from build123d import *

# Parameters (mm, degrees)
F0_R     = 5
F1_DEPTH = 8
F2_W     = 70
F2_H     = 50
F3_DEPTH = 8
F4_W     = 50
F4_H     = 36
F5_DEPTH = 8
F6_R     = 5
F7_DEPTH = 25


with BuildPart() as f1:
    # F0 (on Front) → F1 (new body)
    with BuildSketch(Plane.XZ):
        with BuildLine():
            ThreePointArc((-51.464466, 1.464466), (-49.842349, 0.380602), (-47.928932, 0))
            Line((-47.928932, 0), (50, 0))
            Line((50, 0), (50, 50))
            Line((50, 50), (-47.928932, 50))
            ThreePointArc((-47.928932, 50), (-49.842349, 50.380602), (-51.464466, 51.464466))
            Line((-51.464466, 51.464466), (-71.717587, 71.717587))
            ThreePointArc((-71.717587, 71.717587), (-94.547613, 69.547798), (-96.717812, 46.717812))
            Line((-96.717812, 46.717812), (-51.464466, 1.464466))
        make_face()
        with Locations((-50, 24.999957)):
            Circle(F0_R, mode=Mode.SUBTRACT)
        with Locations((-81.819805, 56.819762)):
            Circle(F0_R, mode=Mode.SUBTRACT)
    extrude(amount=-F1_DEPTH)

    # F2 (on face) → F3 (join)
    with BuildSketch(Plane(origin=(0, 8, 0), x_dir=(-1, 0, 0), z_dir=(0, 1, 0))):
        with Locations((-15, 25)):
            Rectangle(F2_W, F2_H)
    extrude(amount=F3_DEPTH)

    # F4 (on face) → F5 (cut)
    with BuildSketch(Plane(origin=(0, 16, 0), x_dir=(-1, 0, 0), z_dir=(0, 1, 0))):
        with Locations((-25, 25)):
            Rectangle(F4_W, F4_H)
    extrude(amount=-F5_DEPTH, mode=Mode.SUBTRACT)

    # F6 (on face) → F7 (cut)
    with BuildSketch(Plane(origin=(0, 8, 0), x_dir=(-1, 0, 0), z_dir=(0, 1, 0))):
        with Locations((-33, 25)):
            Circle(F6_R)
    extrude(amount=-F7_DEPTH, mode=Mode.SUBTRACT)


solid = f1.part
Could you check a few things on this model? Use its own coordinates, in mm. A direction names the side the tool comes from. Give positions to 0.01 mm unless a question says otherwise; leave off trailing zeros. Write each loop counter-clockwise with the first axis right and the second up, starting at its lowest first coordinate (ties: lowest second). Pieces come first, ordered by that corner, then holes. Notation, with made-up numbers: (-13, 84) -> (40, 84) arc R10 ccw to (40, 101) -> close; hole circle Ø9 at (27, 67.25). An arc over 180 degrees is marked (long way). Answer as a JSON object with one key per item and string values.
Q1. Suppose I cut it at A-A on x = 33. Write out the boundary of the cut face in (y, z).
Taken from the geometry:
{"outline": "(0, 0) -> (16, 0) -> (16, 7) -> (8, 7) -> (8, 20) -> (0, 20) -> close; (0, 30) -> (8, 30) -> (8, 43) -> (16, 43) -> (16, 50) -> (0, 50) -> close"}
Q2. We'd pull the mould along X, two halves only. Please class faces 1 (the flat face through (-20, 12, 25)), 2 (the cylindrical face through (-86.815, 3.944, 57.04)), 3 (the flat face through (25, 8, 25)), 4 (the flat face through (0, 12, 25)): released by +X, released by -X, zero draft, split by the parting line, or undercut.
Taken from the geometry:
{"face 1": "released by -X", "face 2": "undercut", "face 3": "zero draft", "face 4": "released by +X"}
Q3. Suppose I cut it at D-D on z = 22.5. Write out the boundary of the cut face in (x, y).
Taken from the geometry:
{"outline": "(-72.5, 0) -> (-54.33, 0) -> (-54.33, 8) -> (-72.5, 8) -> close; (-45.67, 0) -> (28.67, 0) -> (28.67, 8) -> (0, 8) -> (0, 16) -> (-20, 16) -> (-20, 8) -> (-45.67, 8) -> close; (37.33, 0) -> (50, 0) -> (50, 8) -> (37.33, 8) -> close"}
Q4. Will these pins go through, and if not, where does the flat tip stop? pin 1 Ø4 at (x, y) = (19, 3) entering from +Z; pin 2 Ø11 at (x, z) = (32.5, 26.5) entering from +Y; pin 3 Ø5 at (y, z) = (7.5, 21.5) entering from -X; pin 4 Ø3 at (x, z) = (-32, 52) entering from -Y.
Taken from the geometry:
{"pin 1": "stops at z = 50", "pin 2": "stops at y = 8", "pin 3": "stops at x = -74", "pin 4": "passes through"}
Q5. Suppose I cut it at B-B on z = 33. Write out the boundary of the cut face in (x, y), then the cut area to 3 significant figures.
Taken from the geometry:
{"outline": "(-83, 0) -> (50, 0) -> (50, 8) -> (0, 8) -> (0, 16) -> (-20, 16) -> (-20, 8) -> (-83, 8) -> close", "area": "1,220 mm²"}
Q6. Suppose I cut it at C-C on y = 11.5. Write out the boundary of the cut face in (x, z).
Taken from the geometry:
{"outline": "(-20, 0) -> (50, 0) -> (50, 7) -> (0, 7) -> (0, 43) -> (50, 43) -> (50, 50) -> (-20, 50) -> close"}
Q7. Which directions (+Z, -Z, +X, -X, +Y, -Y) give clear straight access to the entire face, cutting with the end or side of a thin tool? Please do faces 5 (the flat face through (25, 12, 7)), 6 (the cylindrical face through (37, 4, 22)), 7 (the flat face through (13, 8, 50)).
Taken from the geometry:
{"face 5": "+X, +Y", "face 6": "+Y, -Y", "face 7": "+Z, +X, +Y, -Y"}
Q8. Please list where these lines run through material, in increasing order: L1, parallel to Z at x = 23, y = 11; L2, parallel to X at y = 1.25, z = 26; L3, parallel to Z at x = 33, y = 3.25.
Taken from the geometry:
{"L1": "z = 0 to 7, 43 to 50", "L2": "x = -76 to -54.9, -45.1 to 28.1, 37.9 to 50", "L3": "z = 0 to 20, 30 to 50"}
